Could you check a few things on this drawing? It's one solid part, dimensions in mm from its lowest x, y, z. Give positions to 0.01 mm unless a question says otherwise; leave off trailing zeros. Order: outer loops, then holes, each group sorted by start corner. A loop starts at its lowest first (then second) coordinate and runs counter-clockwise, first axis right, second up.
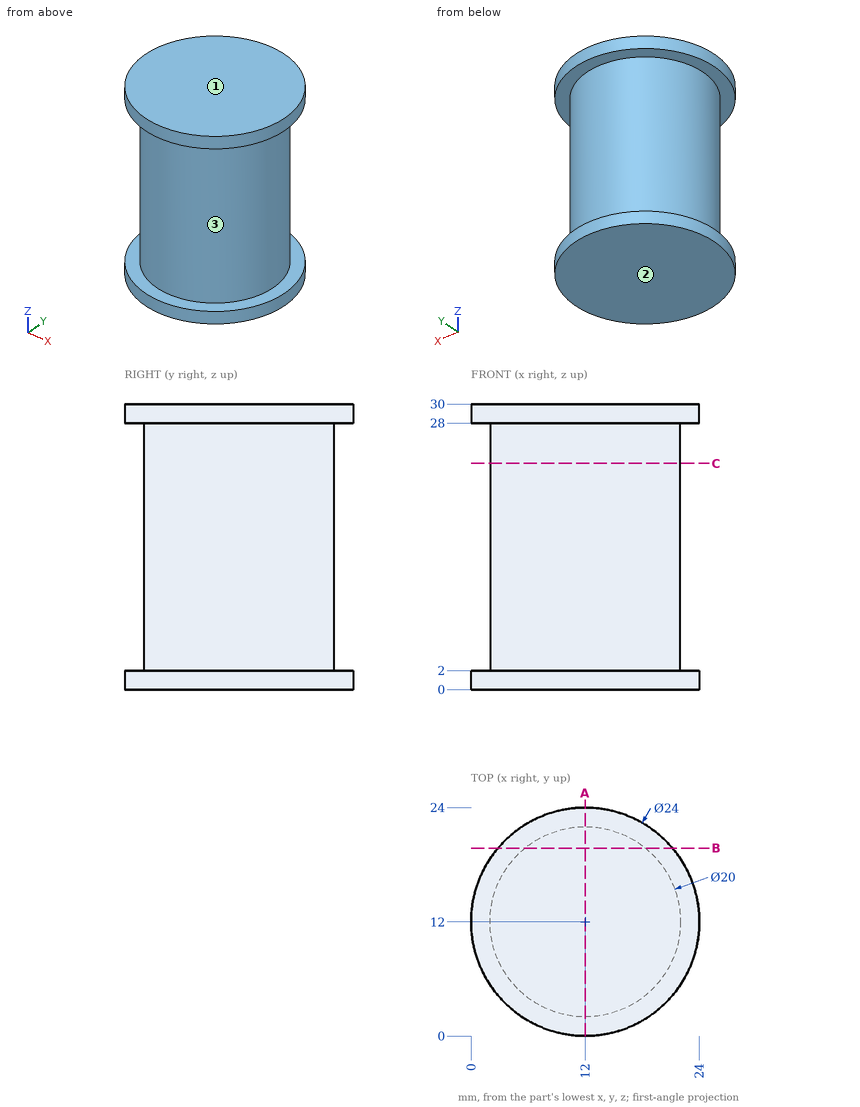
Item 1: Imagine slicing it at C-C on z = 23.75. List the corners of the cut face in (x, y) for me, then the cut area to 3 significant figures.
Findings:
outline: circle Ø20 at (12, 12)
area: 314 mm2
Item 2: Please list where these lines run through material, in increasing order: line 1 along Z through (x, y) = (22.75, 16); line 2 along X through (y, z) = (11.75, 4.25); line 3 along Y through (x, z) = (14.75, 16).
Findings:
line 1: z = 0 to 2, 28 to 30
line 2: x = 2 to 22
line 3: y = 2.39 to 21.61
Item 3: Imagine slicing it at B-B on y = 19.75. List the corners of the cut face in (x, z) for me.
Findings:
outline: (2.84, 0) - (21.16, 0) - (21.16, 2) - (18.32, 2) - (18.32, 28) - (21.16, 28) - (21.16, 30) - (2.84, 30) - (2.84, 28) - (5.68, 28) - (5.68, 2) - (2.84, 2) - close
Item 4: For pin 1 (4 mm diameter, centred on y = 19.5, z = 19, fed in from +X); pin 2 (3 mm diameter, centred on y = 2.5, z = 9.5, fed in from +X); pin 3 (12 mm diameter, centred on y = 6, z = 18, fed in from +X); pin 4 (12 mm diameter, centred on x = 13, y = 8.5, fed in from -Z), each with a flat end and sliding along its axis, tell me the tip position at first contact or that it passes through.
Findings:
pin 1: stops at x = 20.35
pin 2: stops at x = 18
pin 3: stops at x = 22
pin 4: stops at z = 0
Item 5: Imagine slicing it at A-A on x = 12. List the corners of the cut face in (y, z) for me, then the cut area to 3 significant figures.
Findings:
outline: (0, 0) - (24, 0) - (24, 2) - (22, 2) - (22, 28) - (24, 28) - (24, 30) - (0, 30) - (0, 28) - (2, 28) - (2, 2) - (0, 2) - close
area: 616 mm2
Item 6: We'd pull the mould along Z, two halves only. Please class the marked faces 1, 2 and 3: +Z half, -Z half, draft (parallel to the pull), parting line (faces both ways), or undercut.
Findings:
face 1: +Z half
face 2: -Z half
face 3: undercut
